Autodesk Inventor part; units mm, degrees
ref_plane "Work Plane1" through (0, 0, 15) normal (0, 0, 1) x (1, 0, 0)
ref_plane "Work Plane2" through (87.5, 0, 15) normal (-1, 0, 0) x (0, 0, 1)
ref_plane "YZ Plane" through (0, 0, 0) normal (1, 0, 0) x (0, 1, 0)
ref_plane "Work Plane1" through (0, 0, 15) normal (0, 0, 1) x (1, 0, 0)
sketch "Sketch1" plane through (0, 0, 15) normal (0, 0, 1) x (1, 0, 0)
  line L0 (0, 0) -> (175, 0)
  line L1 (175, 0) -> (175, 185)
  line L2 (175, 185) -> (0, 185)
  line L3 (0, 185) -> (0, 0)
  dimension "d7" = 175
  dimension "d8" = 185
extrude "Extrusion1" add sketch "Sketch1" along normal blind 4
sketch "Sketch2" plane through (0, 0, 19) normal (0, 0, 1) x (1, 0, 0)
  line L0 (175, 185) -> (0, 185)
  line L1 (175, 0) -> (175, 185)
  line L2 (0, 185) -> (0, 0)
  point P0 (15.5, 179)
  point P1 (9.5, 167)
  point P2 (21.5, 167)
  point P3 (159.5, 179)
  point P4 (153.5, 167)
  point P5 (165.5, 167)
  dimension "d9" = 12
  dimension "d10" = 6
  dimension "d11" = 6
  dimension "d12" = 12
  dimension "d13" = 6
  dimension "d14" = 12
  dimension "d15" = 6
  dimension "d16" = 12
  dimension "d17" = 6
  dimension "d18" = 6
  dimension "d19" = 144
  dimension "d20" = 9.5
  dimension "d21" = 9.5
hole "Hole1" at (15.5, 179, 19) at (9.5, 167, 19) at (21.5, 167, 19) at (159.5, 179, 19) at (153.5, 167, 19) at (165.5, 167, 19) direction (0, 0, -1) diameter 3.4 end through all
sketch "Sketch3" plane through (0, 0, 19) normal (0, 0, 1) x (1, 0, 0)
  circle A0 centre (153.5, 167) radius 1.7
  circle A1 centre (21.5, 167) radius 1.7
  circle A2 centre (15.5, 179) radius 1.7
  circle A3 centre (9.5, 167) radius 1.7
  circle A4 centre (159.5, 179) radius 1.7
  circle A5 centre (165.5, 167) radius 1.7
  line L0 (175, 0) -> (175, 185)
  line L1 (175, 185) -> (0, 185)
  line L2 (0, 185) -> (0, 0)
  line L3 (0, 0) -> (175, 0)
  line L4 (2, 183) -> (173, 183)
  line L5 (173, 183) -> (173, 2)
  line L6 (173, 2) -> (2, 2)
  line L7 (2, 2) -> (2, 183)
  dimension "d34" = 2
extrude "Extrusion2" add sketch "Sketch3" along normal blind 19.05 contours L3 L2 L1 L0
sketch "Sketch5" plane through (0, 0, 15) normal (0, 0, -1) x (-1, 0, 0)
  line L0 (0, 0) -> (-175, 0)
  line L1 (0, 185) -> (0, 0)
  point P0 (-8.5, 41)
  point P1 (-22.5, 41)
  dimension "d38" = 14
  dimension "d39" = 8.5
  dimension "d40" = 41
sketch "Sketch6" plane through (0, 0, 15) normal (0, -1, 0) x (1, 0, 0)
  line L0 (0, 0) -> (0, 23.05)
  point P0 (0, -15)
  point P1 (8.5, 11.525)
  point P2 (22.5, 11.525)
  point P3 (0, 11.525)
  dimension "d41" = 8.5
  dimension "d42" = 14
hole "Hole2" at (8.5, 41, 15) at (22.5, 41, 15) direction (0, 0, 1) diameter 3 end through all
hole "Hole3" at (8.5, 0, 26.525) at (22.5, 0, 26.525) direction (0, 1, 0) diameter 3 depth 2
ref_plane "Work Plane2" through (87.5, 0, 15) normal (-1, 0, 0) x (0, 0, 1)
mirror "Mirror1" about plane through (87.5, 0, 15) normal (-1, 0, 0) of "Hole2", "Hole3"
sketch "Sketch7" plane through (0, 0, 15) normal (0, -1, 0) x (1, 0, 0)
  line L0 (58.5, 17.5) -> (116.5, 17.5) construction
  line L1 (0, 23.05) -> (175, 23.05) construction
  point P0 (0, -15)
  point P1 (87.5, 17.5)
  point P2 (87.5, 23.05)
  dimension "d57" = 58
  dimension "d58" = 5.55
hole "Hole4" at (58.5, 0, 32.5) at (116.5, 0, 32.5) direction (0, 1, 0) diameter 3 depth 2
sketch "Sketch8" plane through (0, 0, 15) normal (0, 0, -1) x (-1, 0, 0)
  line L0 (0, 0) -> (-175, 0)
  line L1 (-58.5, 10) -> (-116.5, 10) construction
  point P0 (-58.5, 30)
  point P1 (-116.5, 30)
  point P2 (-87.5, 10)
  point P3 (-87.5, 0)
  dimension "d66" = 58
  dimension "d67" = 10
  dimension "d68" = 20
hole "Hole5" at (58.5, 10, 15) at (58.5, 30, 15) at (116.5, 10, 15) at (116.5, 30, 15) direction (0, 0, 1) diameter 3 depth 8
Build history of the part. All positions in model axes, mm. A direction names the side the tool comes from. Coordinates: 2 decimals unless noted, no trailing zeros. Write each loop counter-clockwise with the first axis right and the second up, starting at its lowest first coordinate (ties: lowest second). Pieces come first, ordered by that corner, then holes.
(1) Mould opens along X. For faces 1 (the flat face through (86, 94, 19)), 2 (the flat face through (175, 91, 26)), 3 (the flat face through (86, 94, 15)) say: pulls with the +X half, pulls with the -X half, needs draft (parallel to the pull), parting line crosses it, or undercut.
(2) Pin check, flat tips, straight feed: pin 1 Ø1.8 at (x, z) = (8.5, 26.525) entering from -Y; pin 2 Ø5 at (x, y) = (116.5, 30) entering from +Z. Stop position of each tip, or through.
(3) Drill centre lines: line 1 (X direction, y = 41, z = 16.6); line 2 (X direction, y = 10, z = 16.2); line 3 (X direction, y = 167, z = 16.3). Where is each one in solid material? Low to high.
(4) Cut at B-B on x = 136.5. List the corners of the cut face in (y, z), and give its area (3 significant figures).
(5) Cut at A-A on y = 139.5. List the corners of the cut face in (x, z), and give its area (3 significant figures).
(6) 3-axis set-ups, long thin cutter, end or side, ignore diameter. For faces 4 (the flat face through (86, 183, 28)), 5 (the flat face through (89, 185, 26)): which of +Z, -Z, +X, -X, +Y, -Y reach the whole face in a straight line?
Working result:
1. face 1: undercut
1. face 2: pulls with the +X half
1. face 3: needs draft
2. pin 1: stops at y = 183
2. pin 2: stops at z = 19
3. line 1: x = 0 to 7, 10 to 21, 24 to 151, 154 to 165, 168 to 175
3. line 2: x = 0 to 57, 60 to 115, 118 to 175
3. line 3: x = 0 to 7.8, 11.2 to 19.8, 23.2 to 151.8, 155.2 to 163.8, 167.2 to 175
4. outline: (0, 15) - (185, 15) - (185, 38.05) - (183, 38.05) - (183, 19) - (2, 19) - (2, 38.05) - (0, 38.05) - close
4. area: 816 mm2
5. outline: (0, 15) - (175, 15) - (175, 38.05) - (173, 38.05) - (173, 19) - (2, 19) - (2, 38.05) - (0, 38.05) - close
5. area: 776 mm2
6. face 4: +Z
6. face 5: +Z, -Z, +X, -X, +Y
